Could you check a few things on this model? Use its own coordinates, in mm. Give positions to 0.01 mm unless a question says otherwise; leave off trailing zeros. Order: outer loops, then holes, each group sorted by start corner. A loop starts at its lowest first (then second) coordinate and runs counter-clockwise, first axis right, second up. Notation, with made-up numbers: (66, 84) -> (107, 84) arc R18 cw to (107, 101) -> close; hole circle Ø10 at (22.5, -33.75). An arc over 180 degrees is marked (long way). Write each question's results on one line, items separated by ' | '.
```python
from build123d import *

# Parameters (mm, degrees)
EXTRUDE_1_DEPTH       = 1.6
HOLE_WIZARD_M31_D     = 3.4
HOLE_WIZARD_M31_DEPTH = 10
HOLE_WIZARD_M31_TIP   = 1.021463052


with BuildPart() as part:
    # Эскиз1 → Бобышка-Вытянуть1 (new body)
    with BuildSketch(Plane.XY):
        with BuildLine():
            Line((-16, 34.25), (-16, 41.25))
            Line((-16, 41.25), (16, 41.25))
            Line((16, 41.25), (16, 34.25))
            Line((16, 34.25), (20, 34.25))
            ThreePointArc((20, 34.25), (22.121320344, 33.371320344), (23, 31.25))
            Line((23, 31.25), (23, -31.25))
            ThreePointArc((23, -31.25), (22.121320344, -33.371320344), (20, -34.25))
            Line((20, -34.25), (16, -34.25))
            Line((16, -34.25), (16, -41.25))
            Line((16, -41.25), (-16, -41.25))
            Line((-16, -41.25), (-16, -34.25))
            Line((-16, -34.25), (-20, -34.25))
            ThreePointArc((-20, -34.25), (-22.121320344, -33.371320344), (-23, -31.25))
            Line((-23, -31.25), (-23, 31.25))
            ThreePointArc((-23, 31.25), (-22.121320344, 33.371320344), (-20, 34.25))
            Line((-20, 34.25), (-16, 34.25))
        make_face()
    extrude(amount=EXTRUDE_1_DEPTH)

    # Отверстие с зазором M31
    with Locations(Plane.XY.offset(1.6)):
        with Locations((-19.5, 31), (19.5, 31), (19.5, -31), (-19.5, -31)):
            Hole(HOLE_WIZARD_M31_D / 2, depth=HOLE_WIZARD_M31_DEPTH)
            with Locations((0, 0, -(HOLE_WIZARD_M31_DEPTH + HOLE_WIZARD_M31_TIP / 2))):  # 118° drill point
                Cone(0, HOLE_WIZARD_M31_D / 2, HOLE_WIZARD_M31_TIP, mode=Mode.SUBTRACT)


solid = part.part
```
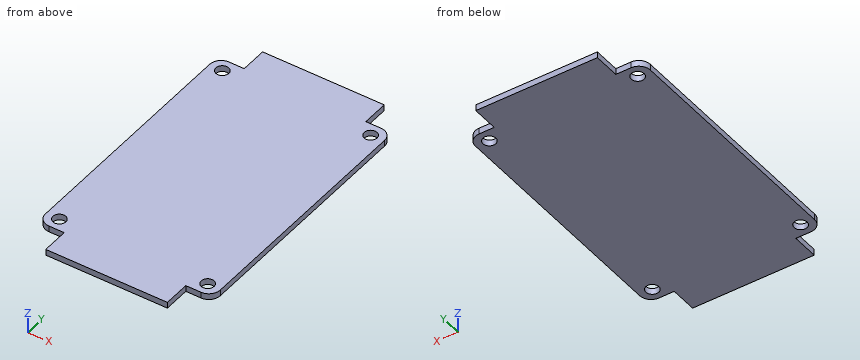
Q1. Suppose I cut it at B-B on y = 36.5. Please give me the cut outline in (x, z).
Here are the results:
outline: (-16, 0) -> (16, 0) -> (16, 1.6) -> (-16, 1.6) -> close
Q2. Suppose I cut it at A-A on z = 0.25. Please give me the cut outline in (x, y).
Here are the results:
outline: (-23, -31.25) arc R3 ccw to (-20, -34.25) -> (-16, -34.25) -> (-16, -41.25) -> (16, -41.25) -> (16, -34.25) -> (20, -34.25) arc R3 ccw to (23, -31.25) -> (23, 31.25) arc R3 ccw to (20, 34.25) -> (16, 34.25) -> (16, 41.25) -> (-16, 41.25) -> (-16, 34.25) -> (-20, 34.25) arc R3 ccw to (-23, 31.25) -> close; hole circle Ø3.4 at (-19.5, -31); hole circle Ø3.4 at (-19.5, 31); hole circle Ø3.4 at (19.5, -31); hole circle Ø3.4 at (19.5, 31)
Q3. I need wall thicknesses on line 1 along Y through (x, z) = (19.5, 0.9); line 2 along Y through (x, z) = (19, 0.3); line 3 along X through (y, z) = (31.5, 1.4). Which ranges of each line are inside material? Lowest first, please.
Here are the results:
line 1: y = -34.25 to -32.7, -29.3 to 29.3, 32.7 to 34.25 | line 2: y = -34.25 to -32.62, -29.38 to 29.38, 32.62 to 34.25 | line 3: x = -22.99 to -21.12, -17.88 to 17.88, 21.12 to 22.99
Q4. I'm going to push flat-ended pins straight in: pin 1 Ø0.8 at (x, z) = (-18.5, 0.5) entering from -Y; pin 2 Ø2 at (x, y) = (-4, -13) entering from -Z; pin 3 Ø0.8 at (x, z) = (-17, 1) entering from +Y; pin 4 Ø0.5 at (y, z) = (39, 0.5) entering from -X. Where does each tip first touch, or does it pass through?
Here are the results:
pin 1: stops at y = -34.25 | pin 2: stops at z = 0 | pin 3: stops at y = 34.25 | pin 4: stops at x = -16
